Read the model definition and answer for the solid it produces. Units are mm, in the model's axes. A direction names the side the tool comes from. Coordinates: 2 decimals unless noted, no trailing zeros. Order: outer loops, then holes, each group sorted by start corner. A loop starts at its lowest first (then second) coordinate and runs counter-clockwise, first axis right, second up. Notation, with made-up numbers: (-15.5, -35) -> (41.5, -35) arc R29 cw to (41.5, -4) -> close; hole circle Ø8 at (-30.5, 50.5). An arc over 180 degrees is marked (long way). Answer as a JSON object with one key per item and string values. Group by question number.
1) Section A-A on z = -12.65 is taken. Determine the outline of the cut face in (x, y).
2) Section C-C on y = 14.8 is taken. Determine the outline of the cut face in (x, z).
3) Section D-D on x = -18 is taken. Determine the outline of the cut face in (y, z).
4) Section B-B on y = 23.5 is taken. Determine the outline of the cut face in (x, z).
5) A tool of negligible diameter and unlimited length cuts with its end or side. For faces 1 (the flat face through (50, 15, -10)), 2 (the flat face through (-48.75, 14, 0)), 3 (the flat face through (-50.75, 14, 0)), from which of +Z, -Z, +X, -X, +Y, -Y can it reach the whole face along a straight path? Write none if from no direction.
6) Given pin 1 (1.6 mm diameter, centred on x = 50, y = 16, fed in from -Z); pin 2 (2 mm diameter, centred on x = 49.5, y = 15.5, fed in from +Z); pin 3 (1 mm diameter, centred on x = 50, z = 1, fed in from -Y), each flat-ended and moving along its own axis, determine where each tip first touches the part or whether it passes through.
7) Consider L1, parallel to X at y = 8.75, z = -2; L2, parallel to Z at x = 34, y = 9.5; L3, parallel to Y at x = 50.25, z = -12.65. Determine where each line is inside the solid, lowest interval first.
8) Determine the mould class of faces 4 (the flat face through (-1, 14, 25.05)), 5 (the cylindrical face through (47.7, 14.2, -22.2)), 6 (the cylindrical face through (48.896, 14.553, -23.095)) for opening direction X: released by +X, released by -X, zero draft, split by the parting line, or undercut.
from build123d import *

# Parameters (mm, degrees)
SKETCH1_W                     = 101.5
SKETCH1_H                     = 50.1
BOSS_EXTRUDE1_DEPTH           = 25.3
FILLET1_R                     = 6.5
FILLET2_R                     = 3.5
CUT_EXTRUDE1_DEPTH            = 23.6
FILLET3_R                     = 1
CUT_EXTRUDE2_REACH            = 107.678
SKETCH3_W                     = 20
SKETCH3_H                     = 11
TAP_DRILL_FOR_4_40_TAP1_D     = 2.2606
TAP_DRILL_FOR_4_40_TAP1_DEPTH = 2
F_1_8_END_MILL_R              = 1.5875


with BuildPart() as part:
    # Sketch1 → Boss-Extrude1 (new body)
    with BuildSketch(Plane(origin=(0, 0, 0), x_dir=(1, 0, 0), z_dir=(0, 1, 0))):
        Rectangle(SKETCH1_W, SKETCH1_H)
    extrude(amount=BOSS_EXTRUDE1_DEPTH)

    # Fillet1
    fillet1_edges = [part.edges().sort_by_distance(p)[0] for p in [
        (50.75, 12.65, 25.05),
        (-50.75, 12.65, 25.05),
        (-50.75, 12.65, -25.05),
        (50.75, 12.65, -25.05),
    ]]
    fillet(fillet1_edges, radius=FILLET1_R)

    # Fillet2
    fillet2_edges = [part.edges().sort_by_distance(p)[0] for p in [
        (-50.75, 0, 0),
        (50.75, 0, 0),
        (0, 0, 25.05),
        (0, 0, -25.05),
        (48.846194078, 0, 23.146194078),
        (-48.846194078, 0, 23.146194078),
        (48.846194078, 0, -23.146194078),
        (-48.846194078, 0, -23.146194078),
    ]]
    fillet(fillet2_edges, radius=FILLET2_R)

    # Sketch2 → Cut-Extrude1 (cut)
    with BuildSketch(Plane(origin=(0, 25.3, 0), x_dir=(1, 0, 0), z_dir=(0, 1, 0))):
        with BuildLine():
            Line((-45.25, 23.2), (45.25, 23.2))
            ThreePointArc((45.25, 23.2), (47.724873734, 22.174873734), (48.75, 19.7))
            Line((48.75, 19.7), (48.75, -19.7))
            ThreePointArc((48.75, -19.7), (47.724873734, -22.174873734), (45.25, -23.2))
            Line((45.25, -23.2), (-45.25, -23.2))
            ThreePointArc((-45.25, -23.2), (-47.724873734, -22.174873734), (-48.75, -19.7))
            Line((-48.75, -19.7), (-48.75, 19.7))
            ThreePointArc((-48.75, 19.7), (-47.724873734, 22.174873734), (-45.25, 23.2))
        make_face()
    extrude(amount=-CUT_EXTRUDE1_DEPTH, mode=Mode.SUBTRACT)

    # Fillet3
    fillet3_edges = [part.edges().sort_by_distance(p)[0] for p in [
        (47.724873734, 1.7, -22.174873734),
        (48.75, 1.7, 0),
        (47.724873734, 1.7, 22.174873734),
        (0, 1.7, 23.2),
        (-47.724873734, 1.7, 22.174873734),
        (-48.75, 1.7, 0),
        (-47.724873734, 1.7, -22.174873734),
        (0, 1.7, -23.2),
    ]]
    fillet(fillet3_edges, radius=FILLET3_R)

    # Sketch3 → Cut-Extrude2 (cut, up to next)
    with BuildSketch(Plane.ZY.offset(-48.75), mode=Mode.PRIVATE) as cut_extrude2_sk1:
        with Locations((0, 14.8)):
            Rectangle(SKETCH3_W, SKETCH3_H)
    cut_extrude2_tool1 = extrude(cut_extrude2_sk1.sketch, amount=-CUT_EXTRUDE2_REACH, mode=Mode.PRIVATE) & part.part
    add(cut_extrude2_tool1.solids().sort_by_distance((48.75, 14.8, 0))[0], mode=Mode.SUBTRACT)

    # Tap Drill for #4-40 Tap1
    with Locations(Plane(origin=(50.75, 0, 0), x_dir=(0, 0, -1), z_dir=(1, 0, 0))):
        with Locations((-12.65, 14.8), (12.65, 14.8)):
            Hole(TAP_DRILL_FOR_4_40_TAP1_D / 2, depth=TAP_DRILL_FOR_4_40_TAP1_DEPTH)

    # 1/8" end mill
    f_1_8_end_mill_edges = [part.edges().sort_by_distance(p)[0] for p in [
        (49.75, 20.3, -10),
        (49.75, 20.3, 10),
        (49.75, 9.3, 10),
        (49.75, 9.3, -10),
    ]]
    fillet(f_1_8_end_mill_edges, radius=F_1_8_END_MILL_R)


solid = part.part
Worked answers:
{
 "1": {"outline": "(-50.75, 3.5) arc R3.5 ccw to (-47.25, 0) -> (47.25, 0) arc R3.5 ccw to (50.75, 3.5) -> (50.75, 13.67) -> (48.75, 13.67) -> (48.75, 2.7) arc R1 cw to (47.75, 1.7) -> (-47.75, 1.7) arc R1 cw to (-48.75, 2.7) -> (-48.75, 25.3) -> (-50.75, 25.3) -> close; (48.75, 15.93) -> (50.75, 15.93) -> (50.75, 25.3) -> (48.75, 25.3) -> close"},
 "2": {"outline": "(-50.75, -18.55) arc R6.5 ccw to (-44.25, -25.05) -> (44.25, -25.05) arc R6.5 ccw to (50.75, -18.55) -> (50.75, -13.78) -> (48.75, -13.78) -> (48.75, -19.7) arc R3.5 cw to (45.25, -23.2) -> (-45.25, -23.2) arc R3.5 cw to (-48.75, -19.7) -> (-48.75, 19.7) arc R3.5 cw to (-45.25, 23.2) -> (45.25, 23.2) arc R3.5 cw to (48.75, 19.7) -> (48.75, 13.78) -> (50.75, 13.78) -> (50.75, 18.55) arc R6.5 ccw to (44.25, 25.05) -> (-44.25, 25.05) arc R6.5 ccw to (-50.75, 18.55) -> close; (48.75, -11.52) -> (50.75, -11.52) -> (50.75, -10) -> (48.75, -10) -> close; (48.75, 10) -> (50.75, 10) -> (50.75, 11.52) -> (48.75, 11.52) -> close"},
 "3": {"outline": "(0, -21.55) arc R3.5 ccw to (3.5, -25.05) -> (25.3, -25.05) -> (25.3, -23.2) -> (2.7, -23.2) arc R1 cw to (1.7, -22.2) -> (1.7, 22.2) arc R1 cw to (2.7, 23.2) -> (25.3, 23.2) -> (25.3, 25.05) -> (3.5, 25.05) arc R3.5 ccw to (0, 21.55) -> close"},
 "4": {"outline": "(-50.75, -18.55) arc R6.5 ccw to (-44.25, -25.05) -> (44.25, -25.05) arc R6.5 ccw to (50.75, -18.55) -> (50.75, 18.55) arc R6.5 ccw to (44.25, 25.05) -> (-44.25, 25.05) arc R6.5 ccw to (-50.75, 18.55) -> close; hole (-48.75, -19.7) arc R3.5 ccw to (-45.25, -23.2) -> (45.25, -23.2) arc R3.5 ccw to (48.75, -19.7) -> (48.75, 19.7) arc R3.5 ccw to (45.25, 23.2) -> (-45.25, 23.2) arc R3.5 ccw to (-48.75, 19.7) -> close"},
 "5": {"face 1": "+X", "face 2": "+Y", "face 3": "+Z, -Z, -X, +Y, -Y"},
 "6": {"pin 1": "stops at z = -22.76", "pin 2": "stops at z = 23.47", "pin 3": "stops at y = 0.82"},
 "7": {"L1": "x = -50.75 to -48.75, 48.75 to 50.75", "L2": "z = -25.05 to -23.2, 23.2 to 25.05", "L3": "y = 1.7 to 13.67, 15.93 to 25.3"},
 "8": {"face 4": "zero draft", "face 5": "undercut", "face 6": "released by +X"}
}
